from build123d import *

# Parameters (mm, degrees)
SKETCH3_R          = 21
SKETCH1_3_R        = 25
SKETCH4_R          = 13
CUT_EXTRUDE2_DEPTH = 81
FILLET2_R          = 1


with BuildPart() as part:
    # Sketch3 → Loft1 section 0
    with BuildSketch(Plane(origin=(0, 85, 0), x_dir=(1, 0, 0), z_dir=(0, 1, 0))):
        Circle(SKETCH3_R)
    # Sketch1<3> → Loft1 section 1
    with BuildSketch(Plane(origin=(0, 0, 0), x_dir=(1, 0, 0), z_dir=(0, 1, 0))):
        Circle(SKETCH1_3_R)
    loft()

    # Sketch4 → Cut-Extrude2 (cut)
    with BuildSketch(Plane(origin=(0, 85, 0), x_dir=(1, 0, 0), z_dir=(0, 1, 0))):
        Circle(SKETCH4_R)
    extrude(amount=-CUT_EXTRUDE2_DEPTH, mode=Mode.SUBTRACT)

    # Fillet2
    fillet2_edges = [part.edges().sort_by_distance(p)[0] for p in [
        (-21, 85, 0),
        (-13, 85, 0),
    ]]
    fillet(fillet2_edges, radius=FILLET2_R)


solid = part.part
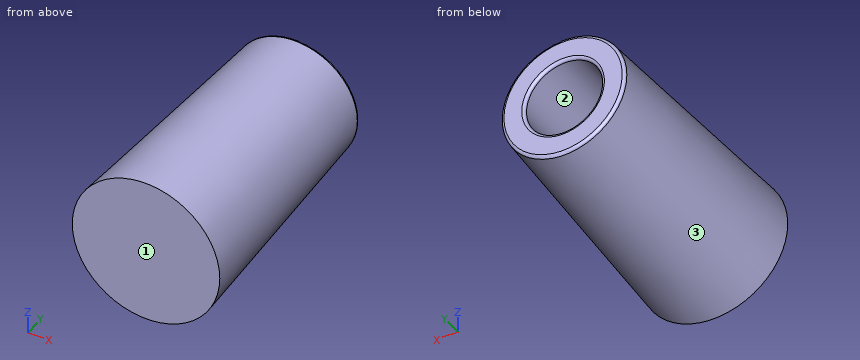
Work out the finished part from the listing and answer in its coordinate system (mm). Face numbers are marked on the shaded views. Round coordinates to 2 decimals unless told otherwise and drop trailing zeros. Loops run counter-clockwise (first coordinate to the right, second up) from the corner with the lowest first, then second, coordinate; pieces in that order, holes last. Notation, with made-up numbers: (80, 66) -> (113, 66) arc R6 cw to (113, 71) -> close; hole circle Ø5 at (58.25, 78.5). An arc over 180 degrees is marked (long way). Use one line per item in the form item = value.
(1) Find section C-C on y = 39. Give the vertices of the cut face in (x, z).
Answer list:
outline = circle Ø46.33 at (0, 0); hole circle Ø26 at (0, 0)
(2) Find section B-B on y = 63. Give the vertices of the cut face in (x, z).
Answer list:
outline = circle Ø44.07 at (0, 0); hole circle Ø26 at (0, 0)
(3) Straight lines are drawn through the part: line 1 (X direction, y = 49, z = -3.5); line 2 (Z direction, x = -12, y = 40); line 3 (Z direction, x = 10.5, y = 19). For each, find the intervals that lie inside material, in ascending order.
Answer list:
line_1 = -22.42 to -12.52, 12.52 to 22.42
line_2 = -19.76 to -5, 5 to 19.76
line_3 = -21.7 to -7.66, 7.66 to 21.7
(4) Find section A-A on x = 0. Give the vertices of the cut face in (y, z).
Answer list:
outline = (0, -25) -> (84.05, -21.04) arc R1 ccw to (85, -20.05) -> (85, -14) arc R1 ccw to (84, -13) -> (4, -13) -> (4, 13) -> (84, 13) arc R1 ccw to (85, 14) -> (85, 20.05) arc R1 ccw to (84.05, 21.04) -> (0, 25) -> close
(5) For a pull along X with two mould halves and no side action, classify the marked faces 1, 2 and 3 as released by +X, released by -X, zero draft, split by the parting line, or undercut.
Answer list:
face_1 = zero draft
face_2 = undercut
face_3 = split by the parting line
(6) Flat-ended cylindrical pins translate along their axes: P1, Ø4, axis at x = -12.5, z = -16, coming from the +Y side; P2, Ø2, axis at y = 49, z = 17, coming from the -X side; P3, Ø8, axis at x = 3.5, z = -4.5, coming from the +Y side; P4, Ø1.5, axis at y = 26, z = -10.5, coming from the -X side. Find the tip coordinate at first contact, or state that the pin passes through.
Answer list:
P1 = 85
P2 = -16.1
P3 = 4
P4 = -21.69
